Job drawing, mm, ordinate dimensions from the low corner. One solid piece. A direction names the side the tool comes from. Round coordinates to 2 decimals unless told otherwise and drop trailing zeros. Loops run counter-clockwise (first coordinate to the right, second up) from the corner with the lowest first, then second, coordinate; pieces in that order, holes last. Notation, with made-up numbers: M 13.5,76 L 24.5,76 A25 cw 24.5,92 Z; hole C 43,34 d10. An arc over 180 degrees is marked long. Use a Markdown table: item, result. Add a question column.
(1) Band-saw the part on B-B, the plane x = 47.5. Write the cut outline in (y, z).
(2) Band-saw the part on C-C, the plane y = 14.75. Write the cut outline in (x, z).
(3) Two-plate mould, pull along X, no slides. Class the marked faces 3, 4 and 5: released by +X, released by -X, zero draft, split by the parting line, or undercut.
(4) Wall check: L1, parallel to X at y = 6.75, z = 17.5; L2, parallel to Y at x = 48.5, z = 18; L3, parallel to X at y = 1.15, z = 10. Give the ranges that are in metal, low to high.
(5) Flat gauge pins, fed straight in: P1, Ø2, axis at y = 6.5, z = 41.5, coming from the -X side; P2, Ø2.5, axis at x = 57.5, y = 1.5, coming from the -Z side; P3, Ø1.1, axis at x = 4, y = 1, coming from the +Z side; P4, Ø5.5, axis at x = 47.5, z = 25, coming from the +Y side. Where does each tip first touch, or does it go through?
(6) Band-saw the part on A-A, the plane x = 32.5. Write the cut outline in (y, z).
(7) Which spindle directions (+Z, -Z, +X, -X, +Y, -Y) get a long thin tool onto all of the face, cutting with end or side? Do the marked faces 1 and 2. Say none if no direction does.
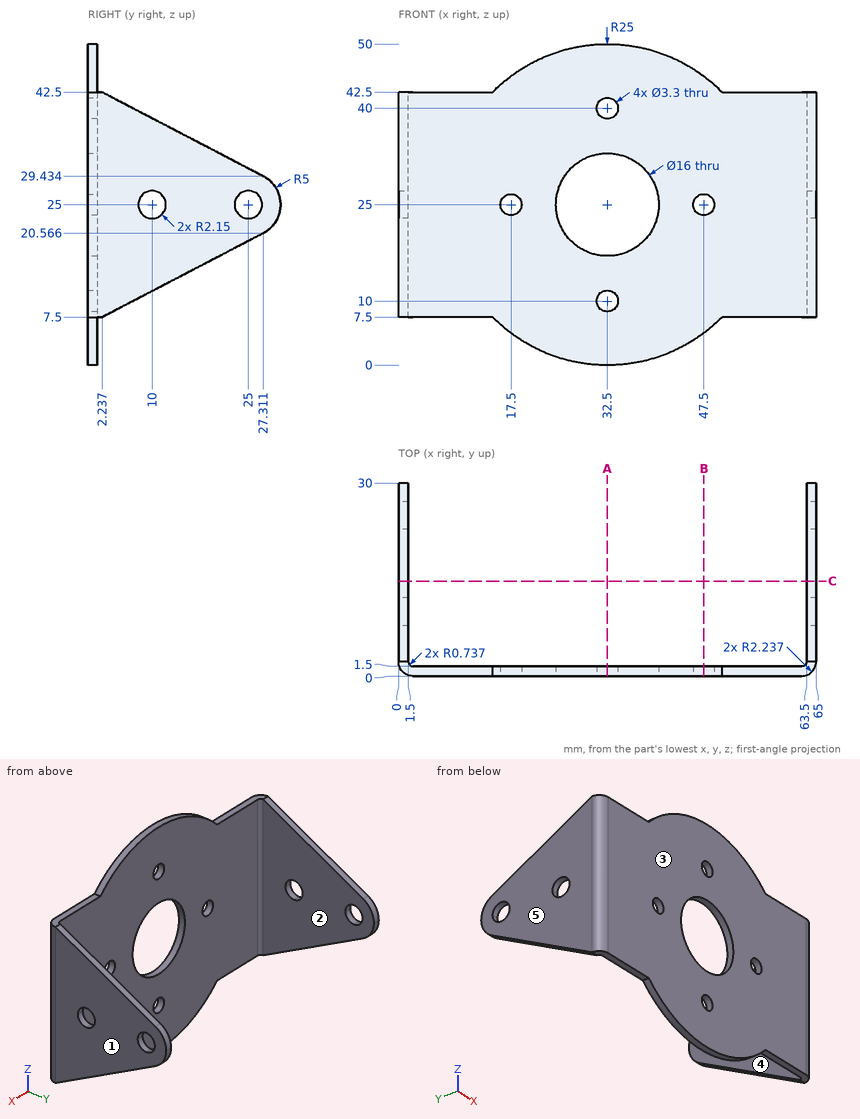
Return value:
| question | item | result |
|---|---|---|
| 1 | outline | M 0,5 L 1.5,5 L 1.5,23.35 L 0,23.35 Z; M 0,26.65 L 1.5,26.65 L 1.5,45 L 0,45 Z |
| 2 | outline | M 0,14.02 L 1.5,14.02 L 1.5,35.98 L 0,35.98 Z; M 63.5,14.02 L 65,14.02 L 65,35.98 L 63.5,35.98 Z |
| 3 | face 3 | zero draft |
| 3 | face 4 | undercut |
| 3 | face 5 | released by -X |
| 4 | L1 | 0 to 1.5, 63.5 to 65 |
| 4 | L2 | 0 to 1.5 |
| 4 | L3 | 0.28 to 30.85, 34.15 to 64.72 |
| 5 | P1 | through |
| 5 | P2 | z = 7.5 |
| 5 | P3 | z = 42.5 |
| 5 | P4 | y = 1.5 |
| 6 | outline | M 0,0 L 1.5,0 L 1.5,8.35 L 0,8.35 Z; M 0,11.65 L 1.5,11.65 L 1.5,17 L 0,17 Z; M 0,33 L 1.5,33 L 1.5,38.35 L 0,38.35 Z; M 0,41.65 L 1.5,41.65 L 1.5,50 L 0,50 Z |
| 7 | face 1 | +Z, -Z, +X, +Y, -Y |
| 7 | face 2 | +Z, -Z, +Y |
